```python
from build123d import *

# Parameters (mm, degrees)
SKETCH1_W           = 234
SKETCH1_H           = 360
BOSS_EXTRUDE1_DEPTH = 6.35
SKETCH2_R           = 2.05
SKETCH2_R_2         = 3.96875
SKETCH2_R_3         = 2.1
CUT_EXTRUDE1_DEPTH  = 10


with BuildPart() as part:
    # Sketch1 → Boss-Extrude1 (new body)
    with BuildSketch(Plane.XY):
        with Locations((3.724430118, 68.459164491)):
            Rectangle(SKETCH1_W, SKETCH1_H)
    extrude(amount=BOSS_EXTRUDE1_DEPTH)

    # Sketch2 → Cut-Extrude1 (cut)
    with BuildSketch(Plane(origin=(0, 0, 0), x_dir=(-1, 0, 0), z_dir=(0, 0, -1))):
        with Locations((107.275569882, -107.540835509)):
            Circle(SKETCH2_R)
        with Locations((107.275569882, -65.540835509)):
            Circle(SKETCH2_R)
        with Locations((41.275569882, -107.540835509)):
            Circle(SKETCH2_R)
        with Locations((41.275569882, -65.540835509)):
            Circle(SKETCH2_R)
        with Locations((29.275569882, -107.540835509)):
            Circle(SKETCH2_R)
        with Locations((29.275569882, -65.540835509)):
            Circle(SKETCH2_R)
        with Locations((-36.724430118, -107.540835509)):
            Circle(SKETCH2_R)
        with Locations((-36.724430118, -65.540835509)):
            Circle(SKETCH2_R)
        with Locations((-48.724430118, -107.540835509)):
            Circle(SKETCH2_R)
        with Locations((-48.724430118, -65.540835509)):
            Circle(SKETCH2_R)
        with Locations((-114.724430118, -107.540835509)):
            Circle(SKETCH2_R)
        with Locations((-114.724430118, -65.540835509)):
            Circle(SKETCH2_R)
        with Locations((10.98704263, 202.255343847)):
            Circle(SKETCH2_R_2)
        with Locations((-110.724430118, -4.879919884)):
            Circle(SKETCH2_R)
        with Locations((103.275569882, -4.879919884)):
            Circle(SKETCH2_R)
        with Locations((103.275569882, 12.120080116)):
            Circle(SKETCH2_R)
        with Locations((-110.724430118, 12.120080116)):
            Circle(SKETCH2_R)
        with Locations((103.275569882, 29.120080116)):
            Circle(SKETCH2_R)
        with Locations((-110.724430118, 29.120080116)):
            Circle(SKETCH2_R)
        with Locations((103.275569882, 46.120080116)):
            Circle(SKETCH2_R)
        with Locations((-110.724430118, 46.120080116)):
            Circle(SKETCH2_R)
        with Locations((103.275569882, 63.120080116)):
            Circle(SKETCH2_R)
        with Locations((-110.724430118, 63.120080116)):
            Circle(SKETCH2_R)
        with Locations((37.682916604, 217.255344198)):
            Circle(SKETCH2_R_3)
        with Locations((51.462268727, 192.880573325)):
            Circle(SKETCH2_R_3)
        with Locations((47.131206773, 127.255344198)):
            Circle(SKETCH2_R_3)
        with Locations((-37.682916604, 217.255344198)):
            Circle(SKETCH2_R_3)
        with Locations((-47.131206773, 127.255344198)):
            Circle(SKETCH2_R_3)
        with Locations((-51.462268727, 192.880573325)):
            Circle(SKETCH2_R_3)
        Polygon((-50.024430118, 248.459164491), (-120.724430118, 123.395497827), (-120.724430118, 248.459164491), align=None)
        Polygon((113.275569882, 248.459164491), (42.575569882, 248.459164491), (113.275569882, 123.395497827), align=None)
    extrude(amount=-CUT_EXTRUDE1_DEPTH, mode=Mode.SUBTRACT)


solid = part.part
```
Can you work these out from the model? Positions are in its coordinate system, mm. Give positions to 0.01 mm unless a question says otherwise; leave off trailing zeros. Order: outer loops, then holes, each group sorted by start corner. A loop starts at its lowest first (then second) coordinate and runs counter-clockwise, first axis right, second up. Notation, with made-up numbers: M 2.25,-20 L 18.25,-20 A22 cw 18.25,7 Z; hole C 0,10.5 d2. An arc over 180 degrees is marked long. Write item = value, one per line. Start each with the question number.
Q1. I need wall thicknesses on probe 1 along Y at (x, z) = (109.5, 3); probe 2 along X at (y, z) = (128.5, 3); probe 3 along Y at (x, z) = (38.5, 3.5). Which ranges of each line are inside material? Lowest first, please. Write a range as [from, to].
Q2. Suppose I cut it at B-B (x = 93). Write out the boundary of the cut face in (y, z), plus the area to 3 significant figures.
Q3. Suppose I cut it at A-A (z = 1.5). Count the separate pieces of the cut face and the enclosed holes in it, plus the area to 3 significant figures.
Q4. We'd pull the mould along X, two halves only. Please class faces 1 (the flat face through (2, 71, 0)), 2 (the flat face through (84.88, 186.8, 3.13)), 3 (the cylindrical face through (-10.47, 206.19, 3.13)): pulls with the +X half, pulls with the -X half, needs draft (parallel to the pull), parting line crosses it, or undercut.
Q5. Suppose I cut it at C-C (x = 61.5). Write out the boundary of the cut face in (y, z).
Check result:
q1.probe_1 = [-111.54, -6.52], [-3.24, 10.48], [13.76, 27.48], [30.76, 44.48], [47.76, 61.48], [64.76, 143.25]
q1.probe_2 = [-110.39, -48.82], [-45.44, 45.44], [48.82, 117.84]
q1.probe_3 = [-111.54, -108.57], [-106.52, -66.57], [-64.52, 215.32], [219.19, 248.46]
q2.outline = M -111.54,0 L 172.44,0 L 172.44,6.35 L -111.54,6.35 Z
q2.area = 1,800 mm2
q3.separate_pieces = 1
q3.enclosed_holes = 29
q3.area = 75,000 mm2
q4.face_1 = needs draft
q4.face_2 = pulls with the +X half
q4.face_3 = undercut
q5.outline = M -111.54,0 L 228.16,0 L 228.16,6.35 L -111.54,6.35 Z
